```python
from build123d import *

# Parameters (mm, degrees)
BOSS_EXTRUDE1_DEPTH = 500
CUT_EXTRUDE1_DEPTH  = 2.375
LPATTERN1_COUNT     = 10
LPATTERN1_PITCH     = 50
FILLET1_R           = 1


with BuildPart() as part:
    # Sketch1 → Boss-Extrude1 (new body)
    with BuildSketch(Plane.XY):
        Polygon((19.5291, 2.375), (0, 2.375), (0, 4.75), (19.5291, 4.75), (20.122, 4.75), (22.497, 2.375), (20.122, 0), (19.5291, 0), align=None)
    extrude(amount=BOSS_EXTRUDE1_DEPTH)

    # Sketch2 → Cut-Extrude1 (cut)
    with BuildSketch(Plane(origin=(0, 4.75, 0), x_dir=(1, 0, 0), z_dir=(0, 1, 0))):
        with BuildLine():
            Line((6.4087, -22.35), (13.1087, -22.35))
            ThreePointArc((13.1087, -22.35), (15.7587, -25), (13.1087, -27.65))
            Line((13.1087, -27.65), (6.4087, -27.65))
            ThreePointArc((6.4087, -27.65), (3.7587, -25), (6.4087, -22.35))
        make_face()
    cut_extrude1 = extrude(amount=-CUT_EXTRUDE1_DEPTH, mode=Mode.SUBTRACT)

    # LPattern1: Cut-Extrude1 ×10
    with Locations(*[(0, 0, i * LPATTERN1_PITCH) for i in range(1, LPATTERN1_COUNT)]):
        add(cut_extrude1, mode=Mode.SUBTRACT)

    # Fillet1
    fillet1_edges = [part.edges().sort_by_distance(p)[0] for p in [
        (22.497, 2.375, 250),
    ]]
    fillet(fillet1_edges, radius=FILLET1_R)


solid = part.part
```
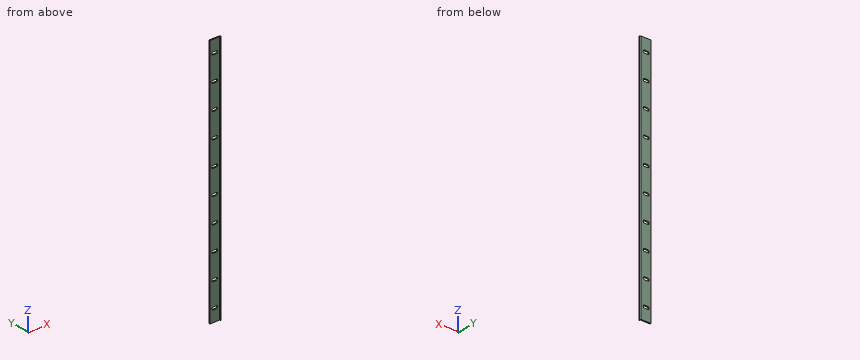
Geometry check sheet. Reference: the model listing, model coordinates, mm. Coordinates: 2 decimals unless noted, no trailing zeros. Loops run counter-clockwise (first coordinate to the right, second up) from the corner with the lowest first, then second, coordinate; pieces in that order, holes last. Notation, with made-up numbers: (55, -30.75) - (107, -30.75) arc R10 cw to (107, -19.75) - close; hole circle Ø2 at (24.5, 26.25). An arc over 180 degrees is marked (long way). One line per item, written item: value. Start each with the question number.
(1) Material ranges on line 1 (Y direction, x = 7.25, z = 348.5) (3 decimals); line 2 (X direction, y = 2.2, z = 366); line 3 (X direction, y = 2.55, z = 266), recorded low to high. Write a range as [from, to].
(2) Depth check by flat-ended pin: P1, Ø0.7, axis at y = 1.5, z = 306.5, coming from the -X side; P2, Ø1, axis at x = 3.5, y = 1.5, coming from the +Z side; P3, Ø4, axis at x = 6, z = 347, coming from the -Y side (3 decimals). Enter the tip coordinate at first touch or a pass-through.
(3) Cross-section at A-A on z = 397. Enter the section's corners in (x, y) (3 decimals), plus the area to 3 significant figures.
Results below:
1. line 1: y = [2.375, 4.75]
1. line 2: x = [19.53, 22.07]
1. line 3: x = [0, 22.07]
2. P1: stops at x = 19.53
2. P2: passes through
2. P3: stops at y = 2.375
3. outline: (0, 2.375) - (19.529, 2.375) - (19.529, 0) - (20.122, 0) - (21.79, 1.668) arc R1 ccw to (21.79, 3.082) - (20.122, 4.75) - (0, 4.75) - close
3. area: 54.6 mm2
